Drawing for the job (mm, zero at the part's lowest x, y, z). A direction names the side the tool comes from. Coordinates: 2 decimals unless noted, no trailing zeros. Loops run counter-clockwise (first coordinate to the right, second up) from the corner with the lowest first, then second, coordinate; pieces in that order, holes last. Notation, with made-up numbers: (18.5, 27.5) -> (48.5, 27.5) arc R36 cw to (48.5, 63.5) -> close; hole circle Ø11 at (66, 8.25). An arc over 180 degrees is marked (long way). Write item = value, one per line. Start each with the question number.
(1) Tool access for the marked faces 1, 2 and 3: list every direction of +Z, -Z, +X, -X, +Y, -Y with a clear straight run to the whole face (end or side of a thin tool).
(2) Band-saw the part on A-A (z = 16.5). Write the cut outline in (x, y).
(3) Band-saw the part on C-C (y = 10.5). Write the cut outline in (x, z).
(4) Drill centre lines: line 1 (X direction, y = 5.75, z = 22.5); line 2 (Y direction, x = 25.5, z = 9.25); line 3 (Z direction, x = 22, y = 22.5). Where is each one in solid material? Low to high. Write a range as from..to.
(5) Band-saw the part on B-B (x = 28). Write the cut outline in (y, z).
(6) Band-saw the part on D-D (z = 8.5). Write the cut outline in (x, y).
(7) Flat gauge pins, fed straight in: P1, Ø6, axis at x = 14, y = 12, coming from the +Z side; P2, Ø4.5, axis at x = 8.5, y = 16, coming from the -Z side. Where does each tip first touch, or does it go through?
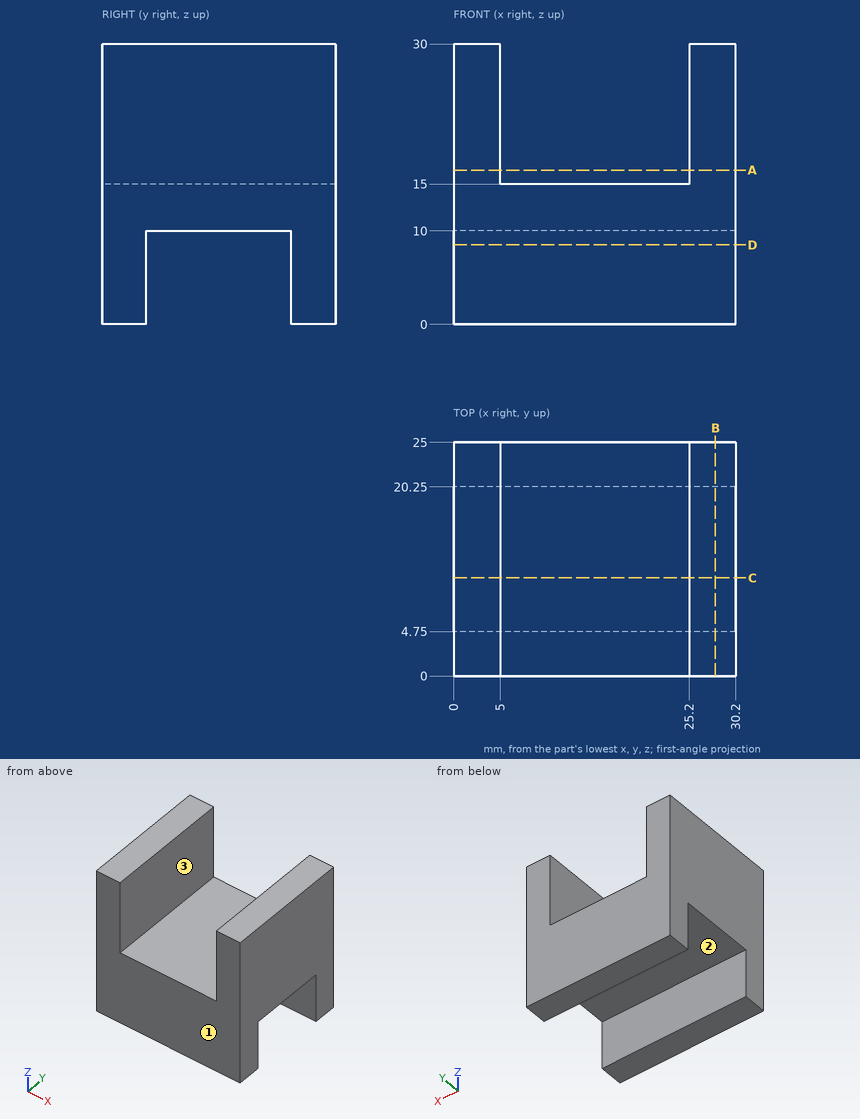
Findings below:
q1.face_1 = +Z, -Z, +X, -X, -Y
q1.face_2 = -Z, +X, -X
q1.face_3 = +Z, +Y, -Y
q2.outline = (0, 0) -> (5, 0) -> (5, 25) -> (0, 25) -> close; (25.2, 0) -> (30.2, 0) -> (30.2, 25) -> (25.2, 25) -> close
q3.outline = (0, 10) -> (30.2, 10) -> (30.2, 30) -> (25.2, 30) -> (25.2, 15) -> (5, 15) -> (5, 30) -> (0, 30) -> close
q4.line_1 = 0..5, 25.2..30.2
q4.line_2 = 0..4.75, 20.25..25
q4.line_3 = 0..15
q5.outline = (0, 0) -> (4.75, 0) -> (4.75, 10) -> (20.25, 10) -> (20.25, 0) -> (25, 0) -> (25, 30) -> (0, 30) -> close
q6.outline = (0, 0) -> (30.2, 0) -> (30.2, 4.75) -> (0, 4.75) -> close; (0, 20.25) -> (30.2, 20.25) -> (30.2, 25) -> (0, 25) -> close
q7.P1 = 15
q7.P2 = 10
